Source: CAD feature listing. Evaluate the final solid. Frame: model axes, mm. A direction names the side the tool comes from. Coordinates: 2 decimals unless noted, no trailing zeros. Write each loop counter-clockwise with the first axis right and the second up, starting at its lowest first coordinate (ties: lowest second). Pieces come first, ordered by that corner, then holes. Notation, with made-up numbers: (28, -36.75) - (36, -36.75) arc R26 cw to (36, -4.75) - close; hole circle Ø8 at (-5, 34). An arc over 180 degrees is marked (long way). One line per item, written item: value.
from build123d import *

# Parameters (mm, degrees)
SKETCH1_R           = 10.3
BOSS_EXTRUDE1_DEPTH = 20.15
BOSS_EXTRUDE2_START = -2.5
SKETCH1_3_R         = 14
SKETCH1_3_R_2       = 10.3
BOSS_EXTRUDE2_DEPTH = 2.5
BOSS_EXTRUDE3_START = -15.85
SKETCH1_4_R         = 10.3
BOSS_EXTRUDE3_DEPTH = 15.85


with BuildPart() as part:
    # Sketch1 → Boss-Extrude1 (new body)
    with BuildSketch(Plane.XY):
        Circle(SKETCH1_R)
    extrude(amount=BOSS_EXTRUDE1_DEPTH)

    # Sketch1_3 → Boss-Extrude2 (add)
    # profile 1 of 2: a face of its own
    with BuildSketch(Plane.XY.offset(BOSS_EXTRUDE2_START)):
        Circle(SKETCH1_3_R)
        Circle(SKETCH1_3_R_2, mode=Mode.SUBTRACT)
    # profile 2 of 2: a face of its own
    with BuildSketch(Plane.XY.offset(BOSS_EXTRUDE2_START)):
        Circle(SKETCH1_3_R_2)
    extrude(amount=BOSS_EXTRUDE2_DEPTH)

    # Sketch1_4 → Boss-Extrude3 (add)
    with BuildSketch(Plane.XY.offset(BOSS_EXTRUDE3_START)):
        Circle(SKETCH1_4_R)
    extrude(amount=BOSS_EXTRUDE3_DEPTH)


solid = part.part
1) Section query A-A on x = 0. Output: boundary loops of the cut face in (y, z), then the cut area to 3 significant figures.
Values found:
outline: (-14, -2.5) - (-10.3, -2.5) - (-10.3, -15.85) - (10.3, -15.85) - (10.3, -2.5) - (14, -2.5) - (14, 0) - (10.3, 0) - (10.3, 20.15) - (-10.3, 20.15) - (-10.3, 0) - (-14, 0) - close
area: 760 mm2
2) Material intervals for line 1 (Z direction, x = 10.5, y = 1.25); line 2 (Y direction, x = -9, z = 14.5); line 3 (Y direction, x = 0.5, z = -2), sorted ascending.
Values found:
line 1: -2.5 to 0
line 2: -5.01 to 5.01
line 3: -13.99 to 13.99
3) Reachability of faces 1 (the cylindrical face through (9.824, 3.094, -9.268)), 2 (the flat face through (0, 0, 20.15)), 3 (the flat face through (-1.1, 10.4, 0)) from +Z, -Z, +X, -X, +Y, -Y: full face, straight path, thin tool, end or side. Return the list, or none.
Values found:
face 1: -Z
face 2: +Z, +X, -X, +Y, -Y
face 3: +Z
4) Contact query for flat-ended pins moving along their axis: P1, Ø4, axis at x = 11, y = 2, coming from the -Z side; P2, Ø1, axis at y = -1, z = -0.5, coming from the -X side; P3, Ø10, axis at y = -4.5, z = 14.5, coming from the -X side; P4, Ø3, axis at x = 10, y = -11, coming from the +Z side. Output: stop coordinate, or through.
Values found:
P1: z = -15.85
P2: x = -13.99
P3: x = -10.3
P4: z = 0
5) Section query C-C on z = 14. Output: boundary loops of the cut face in (x, y).
Values found:
outline: circle Ø20.6 at (0, 0)
